Part model, mm, in its own coordinate system. A direction names the side the tool comes from. Coordinates: 2 decimals unless noted, no trailing zeros. Order: outer loops, then holes, each group sorted by start corner. A loop starts at its lowest first (then second) coordinate and runs counter-clockwise, first axis right, second up. Notation, with made-up numbers: (12.5, -16) - (65.5, -16) arc R16 ccw to (65.5, -11) - close; hole circle Ø3 at (5, 47). An arc over 180 degrees is marked (long way). Use a Markdown table: item, result. Add a question column.
1) Wall check: L1, parallel to X at y = 3.25, z = -27; L2, parallel to X at y = -2.25, z = -24.5; L3, parallel to Z at x = 11, y = -5.25. Give the ranges that are in metal, low to high. Write a range as [from, to].
2) Tool access for faces 1 (the face through (12, -20, 32)), 2 (the face through (29, 3, -27.25)), 3 (the face through (9, -7, 33)), 4 (the face through (-26.23, -4.97, 23.35)), 5 (the face through (-37, -8, -15)): list every direction of +Z, -Z, +X, -X, +Y, -Y with a clear straight run to the whole face (end or side of a thin tool).
3) Drop flat-ended pins along their axis: P1, Ø3.5, axis at x = 6, z = 20, coming from the -Y side; P2, Ø2, axis at y = -4.5, z = -28, coming from the +X side; P3, Ø0.9, axis at y = -13.5, z = 32, coming from the +X side. Give the stop position or say it passes through.
4) Saw through at C-C on y = 1.75. Count the separate pieces of the cut face and the enclosed holes in it, then the cut area to 3 significant figures.
5) Saw through at B-B on x = -23. List the corners of the cut face in (y, z), then the cut area to 3 significant figures.
6) Two-plate mould, pull along X, no slides. Class faces 6 (the face through (26.61, 2.54, -23.14)), 7 (the face through (31.36, -19.1, -31.48)), 8 (the face through (-41.274, 0.809, -26.077)), 9 (the face through (61.73, 1.06, 29.94)): +X half, -X half, draft (parallel to the pull), parting line (faces both ways), or undercut.
7) Saw through at D-D on x = 48.5. List the corners of the cut face in (y, z), then the cut area to 3 significant figures.
8) Saw through at A-A on z = -13. List the corners of the cut face in (x, y).
```python
from build123d import *

# Parameters (mm, degrees)
BOSS_EXTRUDE2_DEPTH     = 3
BOSS_EXTRUDE3_DEPTH     = 20
SKETCH7_R               = 3
SKETCH7_R_2             = 1.75
SKETCH7_R_3             = 2.9
SKETCH7_R_4             = 2.1
BOSS_EXTRUDE4_DEPTH     = 4
SKETCH8_R               = 1.35
CUT_EXTRUDE1_DEPTH      = 66.024995194
SKETCH10_W              = 60
SKETCH10_H              = 3
CUT_EXTRUDE2_DEPTH      = 13
FILLET1_R               = 3
SKETCH11_R              = 1.35
BOSS_EXTRUDE5_DEPTH     = 4
FILLET2_R               = 2
BOSS_EXTRUDE6_START     = 5
BOSS_EXTRUDE6_DEPTH     = 5
SKETCH13_R              = 2
BOSS_EXTRUDE7_DEPTH     = 9.5
SKETCH15_R              = 2
BOSS_EXTRUDE9_DEPTH     = 8
BOSS_EXTRUDE11_DEPTH    = 15.5
CUT_EXTRUDE3_DEPTH      = 74.452365517
CUT_EXTRUDE3_DEPTH_BACK = 74.452365517
FILLET4_R               = 1
FILLET5_R               = 3
BOSS_EXTRUDE12_START    = 1
SKETCH22_R              = 2
BOSS_EXTRUDE12_DEPTH    = 1
SKETCH23_W              = 30
SKETCH23_H              = 3
CUT_EXTRUDE6_DEPTH      = 105.393486418


with BuildPart() as part:
    # Sketch4 → Boss-Extrude2 (new body)
    with BuildSketch(Plane(origin=(0, 0, 0), x_dir=(1, 0, 0), z_dir=(0, 1, 0))):
        with BuildLine():
            Line((49.5, 30), (-29.5, 30))
            ThreePointArc((-29.5, 30), (-33.035533906, 28.535533906), (-34.5, 25))
            Line((-34.5, 25), (-34.5, -25))
            ThreePointArc((-34.5, -25), (-33.035533906, -28.535533906), (-29.5, -30))
            Line((-29.5, -30), (49.5, -30))
            Line((49.5, -30), (54.5, -30))
            Line((54.5, -30), (54.5, -25))
            Line((54.5, -25), (54.5, 25))
            Line((54.5, 25), (54.5, 30))
            Line((54.5, 30), (49.5, 30))
        make_face()
    extrude(amount=-BOSS_EXTRUDE2_DEPTH)

    # Sketch5 → Boss-Extrude3 (add)
    with BuildSketch(Plane(origin=(0, 0, 0), x_dir=(1, 0, 0), z_dir=(0, 1, 0))):
        with BuildLine():
            Line((-29.5, -30), (54.5, -30))
            Line((54.5, -30), (54.5, -33))
            Line((54.5, -33), (-29.5, -33))
            ThreePointArc((-29.5, -33), (-35.156854249, -30.656854249), (-37.5, -25))
            Line((-37.5, -25), (-37.5, 25))
            ThreePointArc((-37.5, 25), (-35.156854249, 30.656854249), (-29.5, 33))
            Line((-29.5, 33), (54.5, 33))
            Line((54.5, 33), (54.5, 30))
            Line((54.5, 30), (-29.5, 30))
            ThreePointArc((-29.5, 30), (-33.035533906, 28.535533906), (-34.5, 25))
            Line((-34.5, 25), (-34.5, -25))
            ThreePointArc((-34.5, -25), (-33.035533906, -28.535533906), (-29.5, -30))
        make_face()
    extrude(amount=-BOSS_EXTRUDE3_DEPTH)

    # Sketch7 → Boss-Extrude4 (add)
    with BuildSketch(Plane.XZ.offset(3)):
        with Locations(Location((-29, -24.5, 0), (0, 0, 90))):
            Circle(SKETCH7_R)
        with Locations(Location((-17.5, -16.4, 0), (0, 0, 90))):
            Circle(SKETCH7_R_2)
        with Locations(Location((29, -24.5, 0), (0, 0, 90))):
            Circle(SKETCH7_R)
        with Locations(Location((34.2, 6.8, 0), (0, 0, 90))):
            Circle(SKETCH7_R_3)
        with Locations(Location((29, 24.5, 0), (0, 0, 90))):
            Circle(SKETCH7_R)
        with Locations(Location((-14, 18.2, 0), (0, 0, 90))):
            Circle(SKETCH7_R_4)
        with BuildLine():
            Line((13.073909236, -10.713655198), (10.223909236, -15.65))
            ThreePointArc((10.223909236, -15.65), (4.35, -17.223909236), (2.776090764, -11.35))
            Line((2.776090764, -11.35), (5.626090764, -6.413655198))
            ThreePointArc((5.626090764, -6.413655198), (11.5, -4.839745962), (13.073909236, -10.713655198))
        make_face()
        with BuildLine():
            Line((5, 6.8), (5, -1.9))
            ThreePointArc((5, -1.9), (3.7, -3.2), (2.4, -1.9))
            Line((2.4, -1.9), (2.4, 6.8))
            ThreePointArc((2.4, 6.8), (3.7, 8.1), (5, 6.8))
        make_face()
        with BuildLine():
            Line((0.5, 20.7), (16.5, 20.7))
            ThreePointArc((16.5, 20.7), (18, 19.2), (16.5, 17.7))
            Line((16.5, 17.7), (0.5, 17.7))
            ThreePointArc((0.5, 17.7), (-1, 19.2), (0.5, 20.7))
        make_face()
        with BuildLine():
            Line((-30.5, 9.9), (-30.5, 21.901923789))
            ThreePointArc((-30.5, 21.901923789), (-29, 27.5), (-27.5, 21.901923789))
            Line((-27.5, 21.901923789), (-27.5, 9.9))
            ThreePointArc((-27.5, 9.9), (-29, 8.4), (-30.5, 9.9))
        make_face()
    extrude(amount=BOSS_EXTRUDE4_DEPTH)

    # Sketch8 → Cut-Extrude1 (cut, through all)
    with BuildSketch(Plane.XZ.offset(7)):
        with Locations(Location((-29, -24.5, 0), (0, 0, 270))):
            Circle(SKETCH8_R)
        with Locations(Location((29, -24.5, 0), (0, 0, 270))):
            Circle(SKETCH8_R)
        with Locations(Location((29, 24.5, 0), (0, 0, 270))):
            Circle(SKETCH8_R)
        with Locations(Location((-29, 24.5, 0), (0, 0, 270))):
            Circle(SKETCH8_R)
    extrude(amount=-CUT_EXTRUDE1_DEPTH, mode=Mode.SUBTRACT)

    # Sketch10 → Cut-Extrude2 (cut)
    with BuildSketch(Plane.XZ.offset(20)):
        with Locations((0.5, -31.5)):
            Rectangle(SKETCH10_W, SKETCH10_H)
    extrude(amount=-CUT_EXTRUDE2_DEPTH, mode=Mode.SUBTRACT)

    # Fillet1
    fillet1_edges = [part.edges().sort_by_distance(p)[0] for p in [
        (-29.5, -7, -31.5),
        (30.5, -7, -31.5),
    ]]
    fillet(fillet1_edges, radius=FILLET1_R)

    # Sketch11 → Boss-Extrude5 (add)
    # profile 1 of 4: a face of its own
    with BuildSketch(Plane.XZ.offset(3)):
        with BuildLine():
            Line((-26, 24.5), (-26, 30))
            Line((-26, 30), (-29.5, 30))
            ThreePointArc((-29.5, 30), (-33.035533906, 28.535533906), (-34.5, 25))
            Line((-34.5, 25), (-34.5, 21.5))
            Line((-34.5, 21.5), (-29, 21.5))
            ThreePointArc((-29, 21.5), (-26.878679656, 22.378679656), (-26, 24.5))
        make_face()
        with Locations(Location((-29, 24.5, 0), (0, 0, 270))):
            Circle(SKETCH11_R, mode=Mode.SUBTRACT)
    # profile 2 of 4: a face of its own
    with BuildSketch(Plane.XZ.offset(3)):
        with BuildLine():
            Line((26, 24.5), (26, 30))
            Line((26, 30), (32, 30))
            Line((32, 30), (32, 24.5))
            ThreePointArc((32, 24.5), (29, 21.5), (26, 24.5))
        make_face()
        with Locations(Location((29, 24.5, 0), (0, 0, 270))):
            Circle(SKETCH11_R, mode=Mode.SUBTRACT)
    # profile 3 of 4: a face of its own
    with BuildSketch(Plane.XZ.offset(3)):
        with BuildLine():
            Line((-29, -21.5), (-34.5, -21.5))
            Line((-34.5, -21.5), (-34.5, -25))
            ThreePointArc((-34.5, -25), (-33.035533906, -28.535533906), (-29.5, -30))
            Line((-29.5, -30), (-26, -30))
            Line((-26, -30), (-26, -24.5))
            ThreePointArc((-26, -24.5), (-26.878679656, -22.378679656), (-29, -21.5))
        make_face()
        with Locations(Location((-29, -24.5, 0), (0, 0, 270))):
            Circle(SKETCH11_R, mode=Mode.SUBTRACT)
    # profile 4 of 4: a face of its own
    with BuildSketch(Plane.XZ.offset(3)):
        with BuildLine():
            Line((26, -24.5), (26, -30))
            Line((26, -30), (32, -30))
            Line((32, -30), (32, -24.5))
            ThreePointArc((32, -24.5), (29, -21.5), (26, -24.5))
        make_face()
        with Locations(Location((29, -24.5, 0), (0, 0, 270))):
            Circle(SKETCH11_R, mode=Mode.SUBTRACT)
    extrude(amount=BOSS_EXTRUDE5_DEPTH)

    # Fillet2
    fillet2_edges = [part.edges().sort_by_distance(p)[0] for p in [
        (-27.5, -5, 21.901923789),
        (-30.5, -5, 21.5),
    ]]
    fillet(fillet2_edges, radius=FILLET2_R)

    # Sketch12 → Boss-Extrude6 (add)
    with BuildSketch(Plane(origin=(0, 0, 0), x_dir=(1, 0, 0), z_dir=(0, 1, 0)).offset(BOSS_EXTRUDE6_START)):
        with BuildLine():
            Line((-29.5, -33), (54.5, -33))
            Line((54.5, -33), (54.5, 33))
            Line((54.5, 33), (-29.5, 33))
            ThreePointArc((-29.5, 33), (-35.156854249, 30.656854249), (-37.5, 25))
            Line((-37.5, 25), (-37.5, -25))
            ThreePointArc((-37.5, -25), (-35.156854249, -30.656854249), (-29.5, -33))
        make_face()
        Polygon((-25.824573519, 24.5), (-27.41228676, 27.25), (-30.58771324, 27.25), (-32.175426481, 24.5), (-30.58771324, 21.75), (-27.41228676, 21.75), align=None, mode=Mode.SUBTRACT)
        Polygon((32.175426481, 24.5), (30.58771324, 27.25), (27.41228676, 27.25), (25.824573519, 24.5), (27.41228676, 21.75), (30.58771324, 21.75), align=None, mode=Mode.SUBTRACT)
        Polygon((32.175426481, -24.5), (30.58771324, -21.75), (27.41228676, -21.75), (25.824573519, -24.5), (27.41228676, -27.25), (30.58771324, -27.25), align=None, mode=Mode.SUBTRACT)
        Polygon((-25.824573519, -24.5), (-27.41228676, -21.75), (-30.58771324, -21.75), (-32.175426481, -24.5), (-30.58771324, -27.25), (-27.41228676, -27.25), align=None, mode=Mode.SUBTRACT)
    extrude(amount=-BOSS_EXTRUDE6_DEPTH)

    # Sketch13 → Boss-Extrude7 (add)
    with BuildSketch(Plane(origin=(0, 5, 0), x_dir=(1, 0, 0), z_dir=(0, 1, 0))):
        with BuildLine():
            Line((-39.5, 33), (-29.5, 33))
            Line((-29.5, 33), (-29.5, 32))
            ThreePointArc((-29.5, 32), (-34.449747468, 29.949747468), (-36.5, 25))
            Line((-36.5, 25), (-36.5, -25))
            ThreePointArc((-36.5, -25), (-34.449747468, -29.949747468), (-29.5, -32))
            Line((-29.5, -32), (-29.5, -33))
            Line((-29.5, -33), (-39.5, -33))
            ThreePointArc((-39.5, -33), (-44.77312059, -29.862551177), (-44.531525851, -23.731399748))
            ThreePointArc((-44.531525851, -23.731399748), (-37.5, 0), (-44.531525851, 23.731399748))
            ThreePointArc((-44.531525851, 23.731399748), (-44.77312059, 29.862551177), (-39.5, 33))
        make_face()
        with Locations(Location((-39.5, 27, 0), (0, 0, 270))):
            Circle(SKETCH13_R, mode=Mode.SUBTRACT)
        with Locations(Location((-39.5, -27, 0), (0, 0, 270))):
            Circle(SKETCH13_R, mode=Mode.SUBTRACT)
    extrude(amount=-BOSS_EXTRUDE7_DEPTH)

    # Sketch15 → Boss-Extrude9 (add)
    with BuildSketch(Plane(origin=(0, 5, 0), x_dir=(1, 0, 0), z_dir=(0, 1, 0))):
        with BuildLine():
            Line((53.5, 33), (53.5, -33))
            Line((53.5, -33), (56.5, -33))
            ThreePointArc((56.5, -33), (61.77312059, -29.862551177), (61.531525851, -23.731399748))
            ThreePointArc((61.531525851, -23.731399748), (54.5, 0), (61.531525851, 23.731399748))
            ThreePointArc((61.531525851, 23.731399748), (61.77312059, 29.862551177), (56.5, 33))
            Line((56.5, 33), (53.5, 33))
        make_face()
        with Locations(Location((56.5, 27, 0), (0, 0, 270))):
            Circle(SKETCH15_R, mode=Mode.SUBTRACT)
        with Locations(Location((56.5, -27, 0), (0, 0, 270))):
            Circle(SKETCH15_R, mode=Mode.SUBTRACT)
    extrude(amount=-BOSS_EXTRUDE9_DEPTH)

    # Sketch19 → Boss-Extrude11 (add)
    with BuildSketch(Plane.XZ.offset(4.5)):
        with BuildLine():
            ThreePointArc((-37.5, 25), (-35.156854249, 30.656854249), (-29.5, 33))
            Line((-29.5, 33), (-39.5, 33))
            ThreePointArc((-39.5, 33), (-44.77312059, 29.862551177), (-44.531525851, 23.731399748))
            ThreePointArc((-44.531525851, 23.731399748), (-39.294857215, 12.375597862), (-37.5, 0))
            Line((-37.5, 0), (-37.5, 25))
        make_face()
        with BuildLine():
            Line((-37.5, -25), (-37.5, 0))
            ThreePointArc((-37.5, 0), (-39.294857215, -12.375597862), (-44.531525851, -23.731399748))
            ThreePointArc((-44.531525851, -23.731399748), (-44.77312059, -29.862551177), (-39.5, -33))
            Line((-39.5, -33), (-29.5, -33))
            ThreePointArc((-29.5, -33), (-35.156854249, -30.656854249), (-37.5, -25))
        make_face()
    extrude(amount=BOSS_EXTRUDE11_DEPTH)

    # Sketch17 → Cut-Extrude3 (cut, two sides: drawn at the far end of the back side and taken through both)
    with BuildSketch(Plane.XY.offset(-CUT_EXTRUDE3_DEPTH_BACK)):
        Polygon((-52.5, 5), (-27.5, -20), (-52.5, -20), align=None)
    extrude(amount=CUT_EXTRUDE3_DEPTH + CUT_EXTRUDE3_DEPTH_BACK, mode=Mode.SUBTRACT)

    # Fillet4
    fillet4_edges = [part.edges().sort_by_distance(p)[0] for p in [
        (-29.5, -18, -31.5),
    ]]
    fillet(fillet4_edges, radius=FILLET4_R)

    # Fillet5
    fillet5_edges = [part.edges().sort_by_distance(p)[0] for p in [
        (30.5, -20, -31.5),
        (54.5, -20, 31.5),
        (54.5, -20, -31.5),
        (-27.5, -20, 31.5),
    ]]
    fillet(fillet5_edges, radius=FILLET5_R)

    # Sketch22 → Boss-Extrude12 (add)
    with BuildSketch(Plane(origin=(0, -4.5, 0), x_dir=(1, 0, 0), z_dir=(0, 1, 0)).offset(BOSS_EXTRUDE12_START)):
        with Locations(Location((-39.5, -27, 0), (0, 0, 270))):
            Circle(SKETCH22_R)
        with Locations(Location((-39.5, 27, 0), (0, 0, 270))):
            Circle(SKETCH22_R)
    extrude(amount=-BOSS_EXTRUDE12_DEPTH)

    # Sketch23 → Cut-Extrude6 (cut, through all)
    with BuildSketch(Plane(origin=(-34.5, 0, 0), x_dir=(0, 0, -1), z_dir=(1, 0, 0))):
        with Locations((0, -8)):
            Rectangle(SKETCH23_W, SKETCH23_H)
    extrude(amount=-CUT_EXTRUDE6_DEPTH, mode=Mode.SUBTRACT)


solid = part.part
```
Results are:
| question | item | result |
|---|---|---|
| 1 | L1 | [-45.5, -41.5], [-37.5, -30.73], [-27.27, 27.27], [30.73, 54.5], [58.5, 62.5] |
| 1 | L2 | [-44.95, -30.35], [-27.65, 27.65], [30.35, 61.95] |
| 1 | L3 | [-33, -30], [-14.31, -4.59], [17.7, 20.7], [30, 33] |
| 2 | face 1 | +Z, -Z, +X, -X, -Y |
| 2 | face 2 | +Y |
| 2 | face 3 | +Z, +X, -X, +Y, -Y |
| 2 | face 4 | -Y |
| 2 | face 5 | -X |
| 3 | P1 | y = -7 |
| 3 | P2 | x = 32 |
| 3 | P3 | x = 54.5 |
| 4 | separate pieces | 1 |
| 4 | enclosed holes | 8 |
| 4 | area | 6,390 mm2 |
| 5 | outline | (-20, 30) - (-3, 30) - (-3, -30) - (-7, -30) - (-7, -33) - (5, -33) - (5, 33) - (-20, 33) - close |
| 5 | area | 591 mm2 |
| 6 | face 6 | undercut |
| 6 | face 7 | -X half |
| 6 | face 8 | undercut |
| 6 | face 9 | +X half |
| 7 | outline | (-20, -33) - (5, -33) - (5, 33) - (-20, 33) - (-20, 30) - (-3, 30) - (-3, -30) - (-20, -30) - close |
| 7 | area | 630 mm2 |
| 8 | outline | (-39.48, -6.5) - (-34.5, -6.5) - (-34.5, -3) - (2.23, -3) - (2.23, -7) - (11.75, -7) - (11.75, -3) - (56.48, -3) - (56.48, 5) - (-39.48, 5) - close; (-38, -9.5) - (-34.5, -13) - (-34.5, -9.5) - close |
